from build123d import *

# Parameters (mm, degrees)
F0_W      = 111.4934720099
F0_H      = 61.2878296524
F1_DEPTH  = 17.78
F2_W      = 111.4934720099
F2_H      = 11.4644090645
F3_DEPTH  = 45.72
F4_W      = 11.9753591716
F4_H      = 49.8234205879
F5_DEPTH  = 35.56
F7_DEPTH  = 25.4
F9_DEPTH  = 25.4
F11_DEPTH = 25.4
F13_DEPTH = 25.4


with BuildPart() as f1:
    # F0 (on Top) → F1 (new body)
    with BuildSketch(Plane.XY):
        with Locations((4.7015305609, -21.1568949744)):
            Rectangle(F0_W, F0_H)
    extrude(amount=F1_DEPTH)

    # F2 (on face) → F3 (join)
    with BuildSketch(Plane.XY.offset(17.78)):
        with Locations((4.7015305609, 3.7548153196)):
            Rectangle(F2_W, F2_H)
    extrude(amount=F3_DEPTH)

    # F4 (on face) → F5 (join)
    with BuildSketch(Plane.XY.offset(17.78)):
        with Locations((-45.0575258583, -26.8890995067)):
            Rectangle(F4_W, F4_H)
    extrude(amount=F5_DEPTH)

    # F6 (on face) → F7 (cut)
    with BuildSketch(Plane.YZ.offset(-39.0698462725)):
        Polygon((-51.8008098006, 27.5652259588), (-26.8890995067, 53.34), (-51.8008098006, 53.34), align=None)
    extrude(amount=-F7_DEPTH, mode=Mode.SUBTRACT)

    # F8 (on face) → F9 (cut)
    with BuildSketch(Plane.XZ.offset(1.9773892127)):
        Polygon((60.4482665658, 63.5), (-4.2021470144, 63.5), (60.4482665658, 32.5463265181), align=None)
    extrude(amount=-F9_DEPTH, mode=Mode.SUBTRACT)

    # F10 (on face) → F11 (cut)
    with BuildSketch(Plane.XY.offset(17.78)):
        Polygon((60.4482665658, -1.9773892127), (7.539015729, -1.9773892127), (-39.0698462725, -51.8008098006), (60.4482665658, -51.8008098006), align=None)
    extrude(amount=-F11_DEPTH, mode=Mode.SUBTRACT)

    # F12 (on face) → F13 (cut)
    with BuildSketch(Plane.XZ.offset(1.9773892127)):
        with BuildLine():
            Line((30.2101253638, 17.603026703), (37.2477211058, 17.603026703))
            Line((37.2477211058, 17.603026703), (37.2477211058, 24.640622445))
            ThreePointArc((37.2477211058, 24.640622445), (32.2713894334, 22.5793583754), (30.2101253638, 17.603026703))
        make_face()
        with BuildLine():
            Line((37.2477211058, 24.640622445), (37.2477211058, 17.603026703))
            Line((37.2477211058, 17.603026703), (44.2853168478, 17.603026703))
            ThreePointArc((44.2853168478, 17.603026703), (42.2240527782, 22.5793583754), (37.2477211058, 24.640622445))
        make_face()
        with BuildLine():
            Line((37.2477211058, 10.565430961), (37.2477211058, 17.603026703))
            Line((37.2477211058, 17.603026703), (30.2101253638, 17.603026703))
            ThreePointArc((30.2101253638, 17.603026703), (32.2713894334, 12.6266950306), (37.2477211058, 10.565430961))
        make_face()
        with BuildLine():
            Line((44.2853168478, 17.603026703), (37.2477211058, 17.603026703))
            Line((37.2477211058, 17.603026703), (37.2477211058, 10.565430961))
            ThreePointArc((37.2477211058, 10.565430961), (42.2240527782, 12.6266950306), (44.2853168478, 17.603026703))
        make_face()
    extrude(amount=-F13_DEPTH, mode=Mode.SUBTRACT)


solid = f1.part
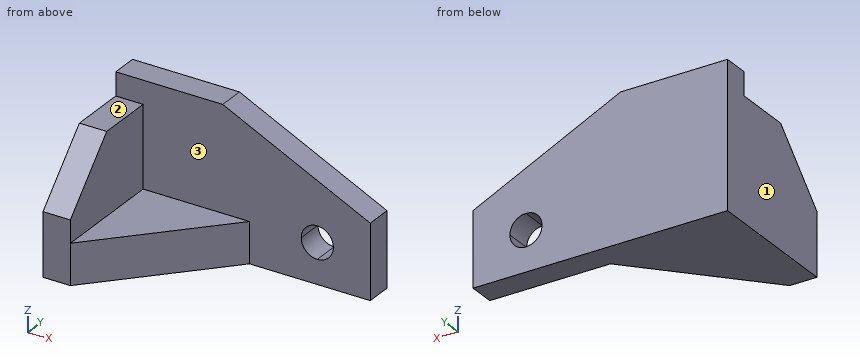
Design review of the part built by this model. Coordinates are the model's own, in mm. Face numbers are marked on the shaded views. A direction names the side the tool comes from. Give positions to 0.01 mm unless a question says otherwise; leave off trailing zeros. Loops run counter-clockwise (first coordinate to the right, second up) from the corner with the lowest first, then second, coordinate; pieces in that order, holes last. Notation, with made-up numbers: M 54,-4.5 L 80,-4.5 A10 cw 80,2.5 Z; hole C -37.75,-39.75 d7. An arc over 180 degrees is marked long. One line per question, with ' | ' between items. Start each with the question number.
1. Add section A-A (y = 0.5). Write out the cut boundary in (x, z), plus the area to 3 significant figures.
2. To check wall thickness, follow L1, parallel to X at y = -23.5, z = 46; L2, parallel to Y at x = 27, z = 40.5; L3, parallel to Z at x = -4, y = -10. State the ranges of each line that lie inside material, in increasing order.
3. Add section B-B (z = 14). Write out the cut boundary in (x, y), plus the area to 3 significant figures.
4. Add section D-D (z = 42). Write out the cut boundary in (x, y), plus the area to 3 significant figures.
5. Add section C-C (y = -13). Write out the cut boundary in (x, z).
6. Insertion check: P1, Ø8, axis at y = -29, z = 24.5, coming from the +X side; P2, Ø4, axis at x = 20, y = -5, coming from the +Z side; P3, Ø14, axis at x = -12.5, y = -31.5, coming from the +Z side; P4, Ø12, axis at y = -8.5, z = 19.5, coming from the +X side. Each pin has a flat end and moves straight along its axis. Give the tip position at first contact, or say it passes through.
7. For the marked faces 1, 2 and 3, list the 3-axis set-ups (+Z, -Z, +X, -X, +Y, -Y) from which the entire face can be reached by the end or side of a thin tool; tool diameter is ignored.
Worked out:
1) outline: M -51.05,0 L 60.45,0 L 60.45,32.55 L -4.2,63.5 L -51.05,63.5 Z; hole C 37.25,17.6 d14.08 | area: 5,920 mm²
2) L1: x = -51.05 to -39.07 | L2: y = -1.98 to 9.49 | L3: z = 0 to 17.78
3) outline: M -51.05,-51.8 L -39.07,-51.8 L 7.54,-1.98 L 31.2,-1.98 L 31.2,9.49 L -51.05,9.49 Z; M 43.29,-1.98 L 60.45,-1.98 L 60.45,9.49 L 43.29,9.49 Z | area: 2,900 mm²
4) outline: M -51.05,-37.85 L -39.07,-37.85 L -39.07,-1.98 L 40.7,-1.98 L 40.7,9.49 L -51.05,9.49 Z | area: 1,480 mm²
5) outline: M -51.05,0 L -2.77,0 L -2.77,17.78 L -39.07,17.78 L -39.07,53.34 L -51.05,53.34 Z
6) P1: stops at x = -39.07 | P2: passes through | P3: stops at z = 17.78 | P4: stops at x = 6.81
7) face 1: +Z, -Z, -X, +Y, -Y | face 2: +Z, +X, -X, -Y | face 3: +Z, +X, -Y
